Part model, mm, in its own coordinate system. A direction names the side the tool comes from. Round coordinates to 2 decimals unless told otherwise and drop trailing zeros. Loops run counter-clockwise (first coordinate to the right, second up) from the corner with the lowest first, then second, coordinate; pieces in that order, holes last. Notation, with made-up numbers: M 59,51 L 115,51 A19 ccw 115,65 Z; hole C 79,-1.75 d2. An arc over 180 degrees is marked long. Write each question's results on one line, items separated by ' | '.
from build123d import *

# Parameters (mm, degrees)
MOVE_FACE1_BY      = 0.075
MOVE_FACE2_BY      = 0.25
SKETCH2_R          = 0.9
CUT_EXTRUDE1_DEPTH = 16.68837149


with BuildPart() as part:
    # Sketch1 → Revolve1 (revolve)
    with BuildSketch(Plane.XY, mode=Mode.PRIVATE) as revolve1_sk:
        Polygon((0, 4), (0, 6.5), (-3, 6.5), (-3, 8.5), (-4, 8.5), (-4, 10.25), (-6, 10.25), (-6, 4), align=None)
    revolve(revolve1_sk.sketch.rotate(Axis((0, 0, 0), (-1, 0, 0)), 90), axis=Axis((0, 0, 0), (-1, 0, 0)))

    # Move Face1: a curved face moved inward by 0.075
    add(Solid.thicken(part.faces().sort_by_distance((-1.5, 0, 6.5))[0], -MOVE_FACE1_BY), mode=Mode.SUBTRACT)

    # Move Face2: a curved face moved inward by 0.25
    add(Solid.thicken(part.faces().sort_by_distance((-3.5, 0, 8.5))[0], -MOVE_FACE2_BY), mode=Mode.SUBTRACT)

    # Sketch2 → Cut-Extrude1 (cut, through all)
    with BuildSketch(Plane.ZY.offset(6)):
        with Locations((0, 8)):
            Circle(SKETCH2_R)
        with Locations((5.656854249, 5.656854249)):
            Circle(SKETCH2_R)
        with Locations((8, 0)):
            Circle(SKETCH2_R)
        with Locations((5.656854249, -5.656854249)):
            Circle(SKETCH2_R)
        with Locations((0, -8)):
            Circle(SKETCH2_R)
        with Locations((-5.656854249, -5.656854249)):
            Circle(SKETCH2_R)
        with Locations((-8, 0)):
            Circle(SKETCH2_R)
        with Locations((-5.656854249, 5.656854249)):
            Circle(SKETCH2_R)
    extrude(amount=-CUT_EXTRUDE1_DEPTH, mode=Mode.SUBTRACT)


solid = part.part
Item 1: Two-plate mould, pull along Z, no slides. Class faces 4 (the cylindrical face through (-1.52, 3.91, 5.1)), 5 (the cylindrical face through (-3.507, 3.127, 7.635)), 6 (the cylindrical face through (-4.85, -7.11, -0.12)): +Z half, -Z half, draft (parallel to the pull), parting line (faces both ways), or undercut.
Filled sheet:
face 4: parting line | face 5: +Z half | face 6: undercut
Item 2: Wall check: L1, parallel to Y at x = -4.9, z = 0; L2, parallel to Y at x = -1.55, z = 0 (3 decimals); L3, parallel to X at y = -7, z = 5. Give the ranges that are in metal, low to high.
Filled sheet:
L1: -10.25 to -8.9, -7.1 to -4, 4 to 7.1, 8.9 to 10.25 | L2: -6.425 to -4, 4 to 6.425 | L3: -6 to -4
Item 3: Drop flat-ended pins along their axis: P1, Ø3, axis at x = -5, y = -3.5, coming from the -Z side; P2, Ø2.5, axis at y = 0, z = 8, coming from the -X side; P3, Ø1.5, axis at x = -1, y = 6.5, coming from the +Z side; P4, Ø1.5, axis at x = -5.5, y = 3.5, coming from the -Z side. Give the stop position or say it passes through.
Filled sheet:
P1: z = -10.05 | P2: x = -6 | P3: z = 2.87 | P4: z = -9.87
Item 4: Band-saw the part on C-C on y = 3. Give the cut face in (x, z), and give its area (3 significant figures).
Filled sheet:
outline: M -6,-9.8 L -4,-9.8 L -4,-7.69 L -3,-7.69 L -3,-5.68 L 0,-5.68 L 0,-2.65 L -6,-2.65 Z; M -6,2.65 L 0,2.65 L 0,5.68 L -3,5.68 L -3,7.69 L -4,7.69 L -4,9.8 L -6,9.8 Z | area: 56.9 mm^2
Item 5: Which spindle directions (+Z, -Z, +X, -X, +Y, -Y) get a long thin tool onto all of the face, cutting with end or side? Do faces 1 (the cylindrical face through (-3.507, 7.635, -3.127)), 2 (the cylindrical face through (-3.507, -7.635, 3.127)), 3 (the cylindrical face through (-3.51, -7.61, -3.19)). Say none if no direction does.
Filled sheet:
face 1: -Z, +X, +Y | face 2: +Z, +X, -Y | face 3: -Z, +X, -Y
Item 6: Band-saw the part on A-A on y = 0. Give the cut face in (x, z) (3 decimals).
Filled sheet:
outline: M -6,-10.25 L -4,-10.25 L -4,-8.9 L -6,-8.9 Z; M -6,-7.1 L -3,-7.1 L -3,-6.425 L 0,-6.425 L 0,-4 L -6,-4 Z; M -6,4 L 0,4 L 0,6.425 L -3,6.425 L -3,7.1 L -6,7.1 Z; M -6,8.9 L -4,8.9 L -4,10.25 L -6,10.25 Z
Item 7: Band-saw the part on D-D on x = -4.75. Count the separate pieces of the cut face and the enclosed holes in it, and give its area (3 significant figures).
Filled sheet:
separate pieces: 1 | enclosed holes: 9 | area: 259 mm^2
